from build123d import *

# Parameters (mm, degrees)
F0_R     = 8
F0_R_2   = 3.5
F1_DEPTH = 2
F2_R     = 6.5
F2_R_2   = 4.75
F3_DEPTH = 3.5
F4_R     = 6.5
F4_R_2   = 5
F5_DEPTH = 3
F6_R     = 6.5
F6_R_2   = 5.25
F7_DEPTH = 3


with BuildPart() as f1:
    # F0 (on Top) → F1 (new body)
    with BuildSketch(Plane.XY):
        Circle(F0_R)
        Circle(F0_R_2, mode=Mode.SUBTRACT)
    extrude(amount=F1_DEPTH)

    # F2 (on face) → F3 (join)
    with BuildSketch(Plane.XY.offset(2)):
        Circle(F2_R)
        Circle(F2_R_2, mode=Mode.SUBTRACT)
    extrude(amount=F3_DEPTH)

    # F4 (on face) → F5 (join)
    with BuildSketch(Plane.XY.offset(5.5)):
        Circle(F4_R)
        Circle(F4_R_2, mode=Mode.SUBTRACT)
    extrude(amount=F5_DEPTH)

    # F6 (on face) → F7 (join)
    with BuildSketch(Plane.XY.offset(8.5)):
        Circle(F6_R)
        Circle(F6_R_2, mode=Mode.SUBTRACT)
    extrude(amount=F7_DEPTH)


solid = f1.part
Model file for the job. Use its own axes, mm. A direction names the side the tool comes from. Coordinates: 2 decimals unless noted, no trailing zeros. Write each loop counter-clockwise with the first axis right and the second up, starting at its lowest first coordinate (ties: lowest second). Pieces come first, ordered by that corner, then holes. Notation, with made-up numbers: (37, 21.5) -> (90, 21.5) arc R8 ccw to (90, 35.5) -> close; hole circle Ø2 at (84.5, 34). An arc over 180 degrees is marked (long way). One line per item, written item: value. Start each with the question number.
1) Slice it at C-C on z = 6. Write the cut outline in (x, y).
2) Flat gauge pins, fed straight in: pin 1 Ø3 at (x, y) = (2, -2) entering from -Z; pin 2 Ø5 at (y, z) = (-6, 3.5) entering from -X; pin 3 Ø1 at (y, z) = (2.5, 6.5) entering from +X; pin 4 Ø3 at (y, z) = (6.5, 8) entering from -X. Where does each tip first touch, or does it go through?
3) Slice it at A-A on x = 0. Write the cut outline in (y, z).
4) Which spindle directions (+Z, -Z, +X, -X, +Y, -Y) get a long thin tool onto all of the face, cutting with end or side? Do faces 1 (the face through (-1.73, -7.81, 0.99)), 2 (the face through (5, 1.6, 10)). Say none if no direction does.
5) Slice it at D-D on x = 6. Write the cut outline in (y, z), then the cut area to 3 significant figures.
6) Pull direction Y, two halves, no side cores. Call faces 3 (the face through (3.4, -1.7, 0)), 4 (the face through (-5.158, -3.955, 6.684)), 5 (the face through (-4, 0, 2)): +Y half, -Y half, draft (parallel to the pull), parting line (faces both ways), or undercut.
7) Probe probe 1 along Y at (x, z) = (0, 7.8); probe 2 along Y at (x, z) = (0, 9.6); probe 3 along Z at (x, y) = (1.75, -4.5). List the from-to ranges inside material, lowest first.
Answers follow:
1. outline: circle Ø13 at (0, 0); hole circle Ø10 at (0, 0)
2. pin 1: z = 0
2. pin 2: x = -6.93
2. pin 3: x = 6.18
2. pin 4: x = -4.15
3. outline: (-8, 0) -> (-3.5, 0) -> (-3.5, 2) -> (-4.75, 2) -> (-4.75, 5.5) -> (-5, 5.5) -> (-5, 8.5) -> (-5.25, 8.5) -> (-5.25, 11.5) -> (-6.5, 11.5) -> (-6.5, 2) -> (-8, 2) -> close; (3.5, 0) -> (8, 0) -> (8, 2) -> (6.5, 2) -> (6.5, 11.5) -> (5.25, 11.5) -> (5.25, 8.5) -> (5, 8.5) -> (5, 5.5) -> (4.75, 5.5) -> (4.75, 2) -> (3.5, 2) -> close
4. face 1: +Z, -Z
4. face 2: +Z
5. outline: (-5.29, 0) -> (5.29, 0) -> (5.29, 2) -> (2.5, 2) -> (2.5, 11.5) -> (-2.5, 11.5) -> (-2.5, 2) -> (-5.29, 2) -> close
5. area: 68.7 mm2
6. face 3: draft
6. face 4: parting line
6. face 5: undercut
7. probe 1: -6.5 to -5, 5 to 6.5
7. probe 2: -6.5 to -5.25, 5.25 to 6.5
7. probe 3: 0 to 5.5
